Check sheet for the drawn part. Datum: minimum x, y, z corner. Units: mm. A direction names the side the tool comes from. Give positions to 0.01 mm unless a question says otherwise; leave off trailing zeros. Order: outer loops, then holes, each group sorted by start corner. A loop starts at its lowest first (then second) coordinate and runs counter-clockwise, first axis right, second up. Notation, with made-up numbers: (76, -33) -> (127, -33) arc R7 cw to (127, -24) -> close; hole circle Ø5 at (24.25, -12). An arc over 180 degrees is marked (long way). Return JSON: item names as keys, results as strings. Group by question number.
(1) Depth check by flat-ended pin: pin 1 Ø1.3 at (y, z) = (1, 1.5) entering from +X; pin 2 Ø0.8 at (x, y) = (13, 9) entering from +Z; pin 3 Ø1.3 at (y, z) = (9, 1.5) entering from -X. Enter the tip coordinate at first touch or a pass-through.
(2) Thickness scan on line 1 along Z through (x, y) = (1, 8.25); line 2 along Y through (x, z) = (7.5, 0.75). Record the ranges inside material, lowest first.
(3) Cross-section at C-C on z = 0.3. Enter the section's corners in (x, y), then the cut area to 3 significant figures.
(4) Cross-section at B-B on x = 9. Enter the section's corners in (y, z), then the cut area to 3 significant figures.
(5) Tool access check on the marked faces 1, 2, 3 and 4. Record the directions out of +Z, -Z, +X, -X, +Y, -Y that give a thin tool (end or side, any length) a straight path to the whole face; none if there is none.
(6) Cross-section at A-A on y = 8.75. Enter the section's corners in (x, z), then the cut area to 3 significant figures.
(7) Cross-section at D-D on x = 2.75. Enter the section's corners in (y, z), then the cut area to 3 significant figures.
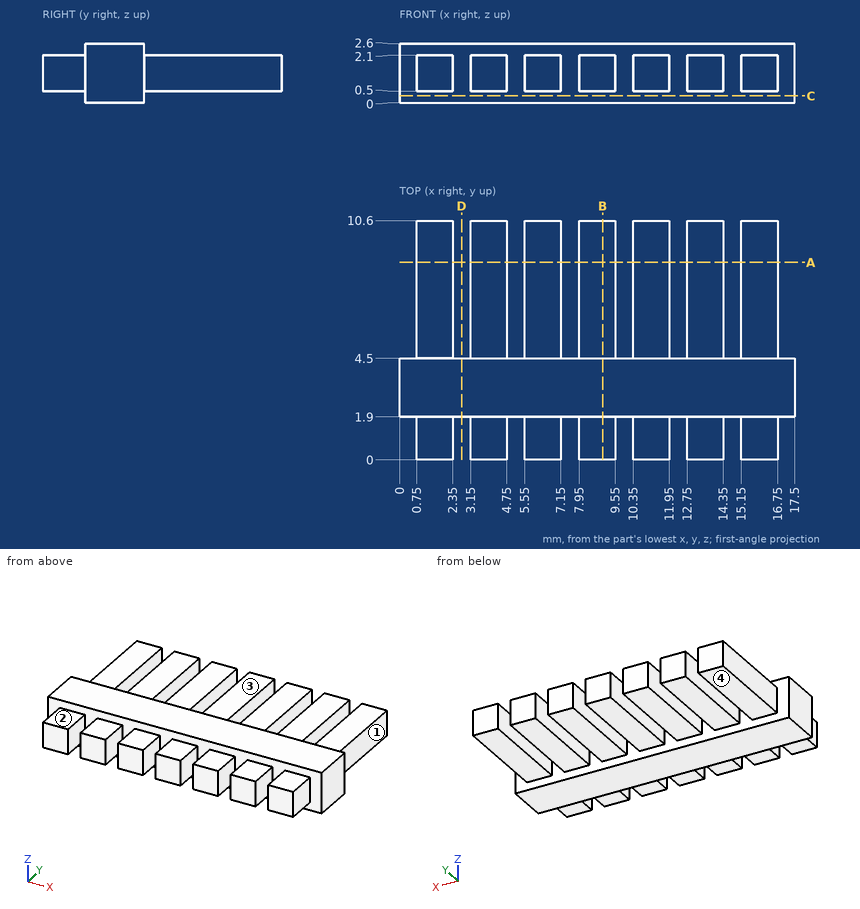
Verdict:
{
 "1": {"pin 1": "x = 16.75", "pin 2": "z = 2.1", "pin 3": "x = 0.75"},
 "2": {"line 1": "0.5 to 2.1", "line 2": "1.9 to 4.5"},
 "3": {"outline": "(0, 1.9) -> (17.5, 1.9) -> (17.5, 4.5) -> (0, 4.5) -> close", "area": "45.5 mm²"},
 "4": {"outline": "(0, 0.5) -> (1.9, 0.5) -> (1.9, 0) -> (4.5, 0) -> (4.5, 0.5) -> (10.6, 0.5) -> (10.6, 2.1) -> (4.5, 2.1) -> (4.5, 2.6) -> (1.9, 2.6) -> (1.9, 2.1) -> (0, 2.1) -> close", "area": "19.6 mm²"},
 "5": {"face 1": "+Z, -Z, +X, +Y", "face 2": "+Z, +X, -X, -Y", "face 3": "+Z, +X, -X, +Y", "face 4": "-Z, +X, -X, +Y"},
 "6": {"outline": "(0.75, 0.5) -> (2.35, 0.5) -> (2.35, 2.1) -> (0.75, 2.1) -> close; (3.15, 0.5) -> (4.75, 0.5) -> (4.75, 2.1) -> (3.15, 2.1) -> close; (5.55, 0.5) -> (7.15, 0.5) -> (7.15, 2.1) -> (5.55, 2.1) -> close; (7.95, 0.5) -> (9.55, 0.5) -> (9.55, 2.1) -> (7.95, 2.1) -> close; (10.35, 0.5) -> (11.95, 0.5) -> (11.95, 2.1) -> (10.35, 2.1) -> close; (12.75, 0.5) -> (14.35, 0.5) -> (14.35, 2.1) -> (12.75, 2.1) -> close; (15.15, 0.5) -> (16.75, 0.5) -> (16.75, 2.1) -> (15.15, 2.1) -> close", "area": "17.9 mm²"},
 "7": {"outline": "(1.9, 0) -> (4.5, 0) -> (4.5, 2.6) -> (1.9, 2.6) -> close", "area": "6.76 mm²"}
}
